Read the model definition and answer for the solid it produces. Units are mm, in the model's axes. A direction names the side the tool comes from. Coordinates: 2 decimals unless noted, no trailing zeros. Loops run counter-clockwise (first coordinate to the right, second up) from the corner with the lowest first, then second, coordinate; pieces in that order, holes last. Notation, with made-up numbers: (69.5, 61) -> (88.5, 61) arc R5 ccw to (88.5, 67) -> close; hole circle Ø11 at (76.5, -9). An arc over 180 degrees is marked (long way). Answer as a JSON object with one key per item and string values. Group by question number.
Q1. The part is cut by section A-A on y = -19. Write down the section's boundary in (x, z).
Q2. Each of these flat-tipped pins is pushed along its axis until it touches: P1, Ø8, axis at y = 21.5, z = 6, coming from the -X side; P2, Ø12, axis at x = 21, y = 12, coming from the -Z side; P3, Ø8, axis at x = 10, z = 1, coming from the -Y side. Where does it stop, or does it pass through?
Q3. The part is cut by section D-D on x = 25.25. Write down the section's boundary in (y, z), and give its area (3 significant figures).
Q4. The part is cut by section C-C on x = 5. Write down the section's boundary in (y, z), and give its area (3 significant figures).
Q5. For faces 1 (the flat face through (10, -15, 10)), 2 (the flat face through (20, 15, 5)), 3 (the flat face through (25, 15, 10)), determine the directions among +Z, -Z, +X, -X, +Y, -Y from which every point of the face is accessible in a straight line to the end or side of a thin tool.
Q6. Straight lines are drawn through the part: line 1 along X through (y, z) = (1.5, 0.25); line 2 along Z through (x, y) = (11, -9); line 3 along Y through (x, z) = (1.75, -0.25). For each, find the intervals that lie inside material, in ascending order. Write a range as [from, to].
Q7. The part is cut by section B-B on z = 7.25. Write down the section's boundary in (x, y), and give its area (3 significant figures).
from build123d import *

# Parameters (mm, degrees)
BOSS_EXTRUDE3_DEPTH = 10
SKETCH5_W           = 30
SKETCH5_H           = 25
BOSS_EXTRUDE5_DEPTH = 5
BOSS_EXTRUDE7_DEPTH = 5


with BuildPart() as part:
    # Sketch3 → Boss-Extrude3 (new body)
    with BuildSketch(Plane.XY):
        Polygon((0, 0), (0, -5), (20, -5), (20, -25), (30, -25), (30, 30), (20, 30), (20, 0), align=None)
    extrude(amount=BOSS_EXTRUDE3_DEPTH)

    # Sketch5 → Boss-Extrude5 (add)
    with BuildSketch(Plane.XY.offset(10)):
        with Locations((15, -12.5)):
            Rectangle(SKETCH5_W, SKETCH5_H)
    extrude(amount=BOSS_EXTRUDE5_DEPTH)

    # Sketch7 → Boss-Extrude7 (add)
    with BuildSketch(Plane(origin=(0, 0, 0), x_dir=(-1, 0, 0), z_dir=(0, 0, -1))):
        Polygon((0, 0), (-20, 0), (-20.758888401, 0), (-30, 0), (-30, -25), (-20, -25), (-20, -5), (0, -5), align=None)
    extrude(amount=BOSS_EXTRUDE7_DEPTH)


solid = part.part
Final values:
{
 "1": {"outline": "(0, 10) -> (20, 10) -> (20, -5) -> (30, -5) -> (30, 15) -> (0, 15) -> close"},
 "2": {"P1": "stops at x = 20", "P2": "stops at z = 0", "P3": "stops at y = -5"},
 "3": {"outline": "(-25, -5) -> (0, -5) -> (0, 0) -> (30, 0) -> (30, 10) -> (0, 10) -> (0, 15) -> (-25, 15) -> close", "area": "800 mm2"},
 "4": {"outline": "(-25, 10) -> (-5, 10) -> (-5, -5) -> (0, -5) -> (0, 15) -> (-25, 15) -> close", "area": "200 mm2"},
 "5": {"face 1": "-Z, -X, -Y", "face 2": "+Z, -Z, -X, +Y", "face 3": "+Z, +X, -X, +Y"},
 "6": {"line 1": "x = [20, 30]", "line 2": "z = [10, 15]", "line 3": "y = [-5, 0]"},
 "7": {"outline": "(0, -5) -> (20, -5) -> (20, -25) -> (30, -25) -> (30, 30) -> (20, 30) -> (20, 0) -> (0, 0) -> close", "area": "650 mm2"}
}
